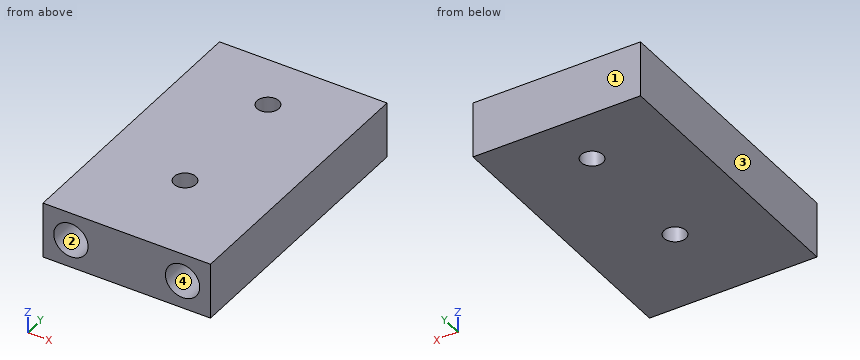
Autodesk Inventor part; units mm, degrees
ref_plane "YZ Plane" through (0, 0, 0) normal (1, 0, 0) x (0, 1, 0)
ref_plane "XZ Plane" through (0, 0, 0) normal (0, 1, 0) x (-1, 0, 0)
ref_plane "XY Plane" through (0, 0, 0) normal (0, 0, 1) x (1, 0, 0)
sketch "Skizze1" plane through (0, 0, 0) normal (0, 0, 1) x (1, 0, 0)
  line L0 (0, 0) -> (12, 0)
  line L1 (12, 0) -> (12, 20)
  line L2 (12, 20) -> (0, 20)
  line L3 (0, 20) -> (0, 0)
  dimension "d0" = 20
  dimension "d1" = 12
extrude "Extrusion1" add sketch "Skizze1" along normal blind 4
sketch "Skizze2" plane through (0, 0, 0) normal (0, -1, 0) x (1, 0, 0)
  line L0 (12, 4) -> (0, 4)
  line L1 (0, 0) -> (0, 4)
  line L2 (0, 0) -> (12, 0)
  line L3 (12, 0) -> (12, 4)
  line L4 (0, 2) -> (12, 2)
  line L5 (6, 4) -> (6, 0)
  point P0 (2, 2)
  point P1 (10, 2)
  dimension "d4" = 8
hole "Bohrung1" at (2, 0, 2) at (10, 0, 2) direction (0, 1, 0) diameter 2.459 depth 10 tip angle 118
sketch "Skizze3" plane through (0, 0, 4) normal (0, 0, 1) x (1, 0, 0)
  line L0 (12, 0) -> (0, 0)
  line L1 (0, 20) -> (12, 20)
  line L2 (6, 0) -> (6, 20)
  point P0 (6, 16)
  point P1 (6, 6.6)
  dimension "d13" = 9.4
  dimension "d14" = 4
hole "Bohrung2" at (6, 16, 4) at (6, 6.6, 4) direction (0, 0, -1) diameter 1.567 depth 10 tip angle 118
properties part number "13_0204_066"
Could you check a few things on this model? Use its own coordinates, in mm. Face numbers are marked on the shaded views. Give positions to 0.01 mm unless a question says otherwise; leave off trailing zeros. Write each loop counter-clockwise with the first axis right and the second up, starting at its lowest first coordinate (ties: lowest second). Pieces come first, ordered by that corner, then holes. Notation, with made-up numbers: (-24.5, 84.25) - (30.5, 84.25) arc R24 ccw to (30.5, 99.25) - close; hole circle Ø5 at (0.5, 8.25). An arc over 180 degrees is marked (long way). One line per item, written item: value. Start each with the question number.
Item 1: I'm going to push flat-ended pins straight in: pin 1 (2 mm diameter, centred on x = 6, y = 6.6, fed in from +Z); pin 2 (2 mm diameter, centred on x = 2, z = 2, fed in from -Y). Where does each tip first touch, or does it pass through?
Item 2: Imagine slicing it at C-C, the plane y = 4.5. List the corners of the cut face in (x, z) for me.
Item 3: Imagine slicing it at B-B, the plane x = 6. List the corners of the cut face in (y, z) for me.
Item 4: If we mould it in two halves opening along X, with no side actions, what happens to the marked faces 1, 2, 3 and 4? For each: +X half, -X half, draft (parallel to the pull), parting line (faces both ways), or undercut.
Item 5: Imagine slicing it at D-D, the plane z = 0.3. List the corners of the cut face in (x, y) for me, and give its area (3 significant figures).
Item 6: Imagine slicing it at A-A, the plane y = 16. List the corners of the cut face in (x, z) for me.
Item 7: Please list where these lines run through material, in increasing order: line 1 (X direction, y = 8.25, z = 2); line 2 (Y direction, x = 6, z = 2.75); line 3 (Y direction, x = 5.75, z = 2.3). Write a range as from..to.
Geometry says:
1. pin 1: z = 4
1. pin 2: y = 10.14
2. outline: (0, 0) - (12, 0) - (12, 4) - (0, 4) - close; hole circle Ø2.46 at (2, 2); hole circle Ø2.46 at (10, 2)
3. outline: (0, 0) - (5.82, 0) - (5.82, 4) - (0, 4) - close; (7.38, 0) - (15.22, 0) - (15.22, 4) - (7.38, 4) - close; (16.78, 0) - (20, 0) - (20, 4) - (16.78, 4) - close
4. face 1: draft
4. face 2: undercut
4. face 3: -X half
4. face 4: undercut
5. outline: (0, 0) - (12, 0) - (12, 20) - (0, 20) - close; hole circle Ø1.57 at (6, 6.6); hole circle Ø1.57 at (6, 16)
5. area: 236 mm^2
6. outline: (0, 0) - (5.22, 0) - (5.22, 4) - (0, 4) - close; (6.78, 0) - (12, 0) - (12, 4) - (6.78, 4) - close
7. line 1: 0..0.77, 3.23..8.77, 11.23..12
7. line 2: 0..5.82, 7.38..15.22, 16.78..20
7. line 3: 0..5.86, 7.34..15.26, 16.74..20
